Could you check a few things on this model? Use its own coordinates, in mm. Give positions to 0.01 mm unless a question says otherwise; leave off trailing zeros. Loops run counter-clockwise (first coordinate to the right, second up) from the corner with the lowest first, then second, coordinate; pieces in that order, holes last. Notation, with made-up numbers: (17.5, 32.5) -> (24.5, 32.5) arc R17 cw to (24.5, 55.5) -> close; hole circle Ø10 at (18.5, 50). An arc over 180 degrees is marked (long way). Put each result on its own line as item: value.
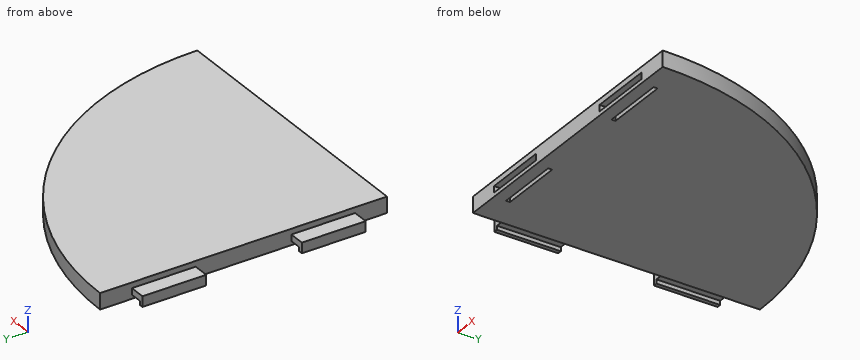
```python
from build123d import *

# Parameters (mm, degrees)
F1_DEPTH = 12.7
F2_W     = 50.8
F2_H     = 5.08
F3_DEPTH = 12.7
F4_W     = 50.8
F4_H     = 5.08
F5_DEPTH = 12.7
F6_W     = 50.8
F6_H     = 3.175
F7_DEPTH = 3.176
F8_W     = 3.175
F8_H     = 50.8
F9_DEPTH = 3.175


with BuildPart() as f1:
    # F0 (on Top) → F1 (new body)
    with BuildSketch(Plane.XY):
        with BuildLine():
            Line((0, 228.6), (0, 0))
            Line((0, 0), (228.6, 0))
            ThreePointArc((228.6, 0), (161.64461, 161.64461), (0, 228.6))
        make_face()
    extrude(amount=F1_DEPTH)

    # F2 (on face) → F3 (cut)
    with BuildSketch(Plane.XZ):
        with Locations((50.8, 5.715)):
            Rectangle(F2_W, F2_H)
        with Locations((177.8, 5.715)):
            Rectangle(F2_W, F2_H)
    extrude(amount=-F3_DEPTH, mode=Mode.SUBTRACT)

    # F4 (on face) → F5 (join)
    with BuildSketch(Plane(origin=(0, 0, 0), x_dir=(0, -1, 0), z_dir=(-1, 0, 0))):
        with Locations((-50.8, 5.715)):
            Rectangle(F4_W, F4_H)
        with Locations((-177.8, 5.715)):
            Rectangle(F4_W, F4_H)
    extrude(amount=F5_DEPTH)

    # F6 (on face) → F7 (cut, through all)
    with BuildSketch(Plane.XY.offset(3.175)):
        with Locations((50.8, 11.1125)):
            Rectangle(F6_W, F6_H)
        with Locations((177.8, 11.1125)):
            Rectangle(F6_W, F6_H)
    extrude(amount=-F7_DEPTH, mode=Mode.SUBTRACT)

    # F8 (on face) → F9 (join)
    with BuildSketch(Plane(origin=(0, 0, 3.175), x_dir=(1, 0, 0), z_dir=(0, 0, -1))):
        with Locations((-11.1125, -177.8)):
            Rectangle(F8_W, F8_H)
        with Locations((-11.1125, -50.8)):
            Rectangle(F8_W, F8_H)
    extrude(amount=F9_DEPTH)


solid = f1.part
```
1. If we section it at C-C (z = 10.75): List the corners of the cut face in (x, y) for me.
Recorded:
outline: (0, 0) -> (228.6, 0) arc R228.6 ccw to (0, 228.6) -> close
2. If we section it at B-B (y = 171.5): List the corners of the cut face in (x, z) for me (3 decimals), then the cut area to 3 significant figures.
Recorded:
outline: (-12.7, 0) -> (-9.525, 0) -> (-9.525, 3.175) -> (0, 3.175) -> (0, 0) -> (151.148, 0) -> (151.148, 12.7) -> (0, 12.7) -> (0, 8.255) -> (-12.7, 8.255) -> close
area: 1,990 mm^2
3. I'm going to push flat-ended pins straight in: pin 1 (4 mm diameter, centred on x = -6, z = 6, fed in from +Y); pin 2 (2.5 mm diameter, centred on x = 186.5, z = 5.5, fed in from -Y); pin 3 (14 mm diameter, centred on x = -9.5, y = 55.5, fed in from +Z) (3 decimals). Where does each tip first touch, or does it pass through?
Recorded:
pin 1: stops at y = 203.2
pin 2: stops at y = 12.7
pin 3: stops at z = 8.255
4. If we section it at D-D (x = 169): List the corners of the cut face in (y, z) for me (3 decimals), then the cut area to 3 significant figures.
Recorded:
outline: (0, 0) -> (9.525, 0) -> (9.525, 3.175) -> (0, 3.175) -> close; (0, 8.255) -> (12.7, 8.255) -> (12.7, 0) -> (153.938, 0) -> (153.938, 12.7) -> (0, 12.7) -> close
area: 1,880 mm^2
5. I need wall thicknesses on line 1 (X direction, y = 47, z = 2.5) (3 decimals); line 2 (X direction, y = 48.5, z = 11); line 3 (Y direction, x = 198, z = 9.5). Which ranges of each line are inside material? Lowest first, please.
Recorded:
line 1: x = -12.7 to -9.525, 0 to 223.716
line 2: x = 0 to 223.4
line 3: y = 0 to 114.25
6. If we section it at A-A (x = 40): List the corners of the cut face in (y, z) for me (3 decimals).
Recorded:
outline: (0, 0) -> (9.525, 0) -> (9.525, 3.175) -> (0, 3.175) -> close; (0, 8.255) -> (12.7, 8.255) -> (12.7, 0) -> (225.073, 0) -> (225.073, 12.7) -> (0, 12.7) -> close
